Read the model definition and answer for the solid it produces. Units are mm, in the model's axes. A direction names the side the tool comes from. Round coordinates to 2 decimals unless told otherwise and drop trailing zeros. Order: outer loops, then holes, each group sorted by start corner. A loop starts at its lowest first (then second) coordinate and runs counter-clockwise, first axis right, second up. Notation, with made-up numbers: (-17, 88) - (-5, 88) arc R22 cw to (-5, 127) - close; hole circle Ø10 at (7.25, 29). An arc over 180 degrees is marked (long way). One line per question, with ' | ' between items. Start each with the question number.
1) The part is cut by section D-D, the plane y = 19. Give the vertices of the cut face in (x, z), plus the area to 3 significant figures.
2) The part is cut by section A-A, the plane x = 15. Give the vertices of the cut face in (y, z) (3 decimals), plus the area to 4 significant figures.
3) The part is cut by section C-C, the plane z = -15.75. Give the vertices of the cut face in (x, y).
4) The mould has two halves that part along Z. Classify faces 1 (the cylindrical face through (50.06, 0.74, -22.39)), 2 (the flat face through (26, 12, 3)), 3 (the cylindrical face through (15, 1, -13)): pulls with the +Z half, pulls with the -Z half, needs draft (parallel to the pull), parting line crosses it, or undercut.
5) Straight lines are drawn through the part: line 1 (Z direction, x = 49, y = 1.05); line 2 (Y direction, x = 2.3, z = -21); line 3 (Z direction, x = 49, y = 2.3). For each, find the intervals that lie inside material, in ascending order. Write a range as from..to.
6) The part is cut by section B-B, the plane y = 13. Give the vertices of the cut face in (x, z) (3 decimals).
7) Flat-ended cylindrical pins translate along their axes: pin 1 (6.5 mm diameter, centred on x = 31, y = 13.5, fed in from -Z); pin 2 (5 mm diameter, centred on x = 49, z = -21, fed in from +Y); pin 3 (3.5 mm diameter, centred on x = 27.5, z = -18, fed in from +Y). Find the tip coordinate at first contact, or state that the pin passes through.
8) For faces 4 (the cylindrical face through (40.6, 1, -12.7)), 5 (the cylindrical face through (2.2, 20.8, -18.6)), 6 (the flat face through (53, 2, -7)), 7 (the flat face through (51, 1.5, -21)), 8 (the flat face through (28, 3, -12)), determine the directions among +Z, -Z, +X, -X, +Y, -Y from which every point of the face is accessible in a straight line to the end or side of a thin tool.
Autodesk Inventor part; units mm, degrees
ref_plane "YZ Plane" through (0, 0, 0) normal (1, 0, 0) x (0, 1, 0)
ref_plane "XZ Plane" through (0, 0, 0) normal (0, 1, 0) x (-1, 0, 0)
ref_plane "XY Plane" through (0, 0, 0) normal (0, 0, 1) x (1, 0, 0)
sketch "Skizze1" plane through (0, 0, 0) normal (0, 0, 1) x (1, 0, 0)
  line L0 (0, 0) -> (53, 0)
  line L1 (53, 0) -> (53, 23)
  line L2 (53, 23) -> (0, 23)
  line L3 (0, 23) -> (0, 0)
  circle A0 centre (15, 13) radius 8.375
  circle A1 centre (40.5, 13) radius 8.375
  dimension "D" = 16.75
  dimension "d1" = 16.75
  dimension "Hoehe" = 23
  dimension "L" = 53
  dimension "d5" = 15
  dimension "d7" = 10
  dimension "d14" = 12.5
extrude "Extrusion1" add sketch "Skizze1" along normal blind 3
sketch "Skizze2" plane through (0, 0, 0) normal (0, 0, -1) x (-1, 0, 0)
  line L0 (-53, 0) -> (-53, 23)
  line L1 (0, 0) -> (-53, 0)
  line L2 (0, 23) -> (0, 0)
  line L3 (-53, 23) -> (0, 23)
  circle A0 centre (-15, 13) radius 8.375
  circle A1 centre (-40.5, 13) radius 8.375
  line L4 (-53, 23) -> (0, 23)
  line L5 (-3, 23) -> (-3, 3)
  line L6 (-3, 3) -> (-53, 3)
  dimension "Dicke" = 3
  dimension "d11" = 3
extrude "Extrusion2" add sketch "Skizze2" along normal blind 25 contours L0 L6 L5 L3 L2 L1
sketch "Skizze3" plane through (3, 3, 0) normal (0, 1, 0) x (1, 0, 0)
  line L0 (50, 0) -> (50, 25)
  line L1 (0, 25) -> (50, 25)
  point P0 (-3, 0)
  point P1 (46, 21)
  dimension "d22" = 4
  dimension "d23" = 4
hole "Bohrung1" at (49, 3, -21) direction (0, -1, 0) diameter 3.5 end through all counterbore diameter 6 counterbore depth 1.5
sketch "Skizze4" plane through (3, 3, 0) normal (1, 0, 0) x (0, 0, -1)
  line L0 (0, 20) -> (25, 20)
  line L1 (25, 20) -> (25, 0)
  point P0 (0, -3)
  point P1 (21, 16)
  dimension "d31" = 4
  dimension "d32" = 4
hole "Bohrung2" at (3, 19, -21) direction (-1, 0, 0) diameter 3.5 end through all counterbore diameter 6 counterbore depth 1.5
sketch "Skizze5" plane through (0, 0, -25) normal (0, 0, -1) x (-1, 0, 0)
  circle A0 centre (-40.5, 13) radius 8.375
  circle A1 centre (-15, 13) radius 8.375
  circle A2 centre (-40.5, 13) radius 12
  circle A3 centre (-15, 13) radius 12
  point P0 (0, 0)
  point P1 (-29.75, 9.4628)
  point P2 (-29.75, 14.5372)
  dimension "d33" = 24
  dimension "d34" = 24
extrude "Extrusion3" cut sketch "Skizze5" against normal blind 25
equation "\"d1\" = D"
equation "\"d11\" = Dicke"
equation "\"d34\" = d33"
properties part number "Buttons_Mount_v3"
Values:
1) outline: (0, -25) - (3, -25) - (3, -24) - (1.5, -24) - (1.5, -22.75) - (0, -22.75) - close; (0, -19.25) - (1.5, -19.25) - (1.5, -18) - (3, -18) - (3, 0) - (9.16, 0) - (9.16, 3) - (0, 3) - close; (20.84, 0) - (34.66, 0) - (34.66, 3) - (20.84, 3) - close; (46.34, 0) - (53, 0) - (53, 3) - (46.34, 3) - close | area: 150 mm^2
2) outline: (0, -25) - (1, -25) - (1, 0) - (4.625, 0) - (4.625, 3) - (0, 3) - close; (21.375, 0) - (23, 0) - (23, 3) - (21.375, 3) - close | area: 43.75 mm^2
3) outline: (0, 0) - (53, 0) - (53, 3) - (47.13, 3) arc R12 cw to (33.87, 3) - (21.63, 3) arc R12 cw to (8.37, 3) - (3, 3) - (3, 23) - (0, 23) - close
4) face 1: undercut | face 2: pulls with the +Z half | face 3: needs draft
5) line 1: z = -25..-22.75, -19.25..3 | line 2: y = 0..16, 22..23 | line 3: z = -25..-24, -18..3
6) outline: (0, -25) - (3, -25) - (3, 0) - (6.625, 0) - (6.625, 3) - (0, 3) - close; (23.375, 0) - (32.125, 0) - (32.125, 3) - (23.375, 3) - close; (48.875, 0) - (53, 0) - (53, 3) - (48.875, 3) - close
7) pin 1: stops at z = 0 | pin 2: stops at y = 1.5 | pin 3: stops at y = 3
8) face 4: -Z, +Y | face 5: +X | face 6: +Z, -Z, +X, +Y, -Y | face 7: +Y | face 8: -Z, +X, +Y
